Source: CAD feature listing. Evaluate the final solid. Frame: model axes, mm. A direction names the side the tool comes from. Coordinates: 2 decimals unless noted, no trailing zeros. Loops run counter-clockwise (first coordinate to the right, second up) from the corner with the lowest first, then second, coordinate; pieces in that order, holes last.
```python
from build123d import *

# Parameters (mm, degrees)
BOSS_EXTRUDE1_DEPTH = 15
SKETCH2_R           = 1.5
BOSS_EXTRUDE2_DEPTH = 4
SKETCH3_R           = 1.5
BOSS_EXTRUDE3_DEPTH = 4


with BuildPart() as part:
    # Sketch1 → Boss-Extrude1 (new body)
    with BuildSketch(Plane(origin=(0, 0, 0), x_dir=(1, 0, 0), z_dir=(0, 1, 0))):
        Polygon((1.800179217, -1.569235172), (2.259087132, 0.774383347), (0.458907915, 2.343618519), (-1.800179217, 1.569235172), (-2.259087132, -0.774383347), (-0.458907915, -2.343618519), align=None)
    extrude(amount=BOSS_EXTRUDE1_DEPTH)

    # Sketch2 → Boss-Extrude2 (add)
    with BuildSketch(Plane(origin=(0, 15, 0), x_dir=(1, 0, 0), z_dir=(0, 1, 0))):
        Circle(SKETCH2_R)
    extrude(amount=BOSS_EXTRUDE2_DEPTH)

    # Sketch3 → Boss-Extrude3 (add)
    with BuildSketch(Plane.XZ):
        Circle(SKETCH3_R)
    extrude(amount=BOSS_EXTRUDE3_DEPTH)


solid = part.part
```
Q1. First-contact query: pin 1 Ø1.5 at (x, y) = (1.5, 15.5) entering from -Z. Flat tip, straight axial feed; report the tip coordinate or a pass-through.
Q2. Reachability of faces 1 (the flat face through (0, 15, 2)), 2 (the flat face through (1.37, 7.4, -1.55)), 3 (the flat face through (0, 0, 2)) from +Z, -Z, +X, -X, +Y, -Y: full face, straight path, thin tool, end or side. Return the list, or none.
Q3. Section query D-D on y = -0.5. Return the cut outline in (x, z).
Q4. Material intervals for line 1 along Y through (x, z) = (-1.5, 0.6); line 2 along X through (y, z) = (15.75, 0); line 3 along X through (y, z) = (2.5, 0.8), sorted ascending.
Q5. Section query B-B on z = -0.2. Return the cut outline in (x, y), then the cut area to 3 significant figures.
Q6. Section query A-A on y = 14.5. Return the cut outline in (x, z), then the cut area to 3 significant figures.
Q7. Section query C-C on x = 1.3. Return the cut outline in (y, z), then the cut area to 3 significant figures.
Resolved:
1. pin 1: stops at z = -1.92
2. face 1: +Y
2. face 2: -Z, +X, +Y, -Y
2. face 3: -Y
3. outline: circle Ø3 at (0, 0)
4. line 1: y = 0 to 15
4. line 2: x = -1.5 to 1.5
4. line 3: x = -2.23 to 1.95
5. outline: (-2.07, 0) - (-1.49, 0) - (-1.49, -4) - (1.49, -4) - (1.49, 0) - (2.15, 0) - (2.15, 15) - (1.49, 15) - (1.49, 19) - (-1.49, 19) - (-1.49, 15) - (-2.07, 15) - close
5. area: 87.0 mm2
6. outline: (-2.26, 0.77) - (-1.8, -1.57) - (0.46, -2.34) - (2.26, -0.77) - (1.8, 1.57) - (-0.46, 2.34) - close
6. area: 14.8 mm2
7. outline: (-4, -0.75) - (0, -0.75) - (0, -1.61) - (15, -1.61) - (15, -0.75) - (19, -0.75) - (19, 0.75) - (15, 0.75) - (15, 1.74) - (0, 1.74) - (0, 0.75) - (-4, 0.75) - close
7. area: 62.2 mm2
